Part model, mm, in its own coordinate system. Coordinates: 2 decimals unless noted, no trailing zeros. Loops run counter-clockwise (first coordinate to the right, second up) from the corner with the lowest first, then second, coordinate; pieces in that order, holes last. Notation, with made-up numbers: M -32,70 L 21,70 A30 cw 21,94 Z; hole C 9,36.5 d9. An arc over 180 degrees is marked long. Use a Markdown table: item, result. Add a question column.
1) Band-saw the part on C-C (x = -10.5). List the corners of the cut face in (y, z).
2) Band-saw the part on B-B (y = 0.5). List the corners of the cut face in (x, z), plus the area to 3 significant figures.
3) Pin check, flat tips, straight feed: pin 1 Ø1 at (y, z) = (0, 14.5) entering from +X; pin 2 Ø10 at (x, z) = (11, 5) entering from -Y; pin 3 Ø6 at (x, y) = (1, 8.5) entering from +Z. Stop position of each tip, or through.
4) Band-saw the part on A-A (z = 5). List the corners of the cut face in (x, y) (1 decimal).
5) Wall check: probe 1 along Y at (x, z) = (-1, 4); probe 2 along X at (y, z) = (-6, 3.5); probe 3 along Y at (x, z) = (-7.5, 13.25). Give the ranges that are in metal, low to high. Write a range as from..to.
6) Band-saw the part on D-D (z = 1.5). List the corners of the cut face in (x, y), plus the area to 3 significant figures.
Autodesk Fusion 360 part; units mm, degrees
sketch "草图1" plane through (0, 0, 0) normal (0, 1, 0) x (1, 0, 0)
  line L0 (0, -55) -> (0, 50) construction
  line L1 (-125, 0) -> (125, 0) construction
  line L2 (-31, 0) -> (20, 0)
  circle A0 centre (20, -1) radius 1
  arc A1 (-31.065, -5.889) -> (18.5199, -10.8983) centre (-3, 24) ccw
  line L3 (-31.6884, -4.6053) -> (-31.9962, -1.0872)
  line L4 (20.4052, -7.8422) -> (20.9962, -1.0872)
  line L5 (21, 0) -> (21, -0.6) construction
  line L6 (-32, 0) -> (-32, -0.7) construction
  line L7 (0, -17) -> (10, -17) construction
  arc A2 (-31, 0) -> (-31.9962, -1.0872) centre (-31, -1) ccw
  arc A3 (-31.6884, -4.6053) -> (-31.065, -5.889) centre (-29.696, -4.431) ccw
  arc A4 (-8, 0) -> (8, 0) centre (0, 0) ccw
  arc A5 (18.5199, -10.8983) -> (20.4052, -7.8422) centre (16.4204, -7.4936) ccw
  line L8 (0, -8) -> (0, 0)
  dimension "d1" = 16
  dimension "d2" = 2
  dimension "d3" = 2
  dimension "d4" = 5
  dimension "d5" = 5
  dimension "d6" = 8
  dimension "d7" = 4
  dimension "d8" = 21
  dimension "d9" = 53
  dimension "d10" = 41
  dimension "d11" = 17
  dimension "d12" = 24
  dimension "d13" = 24
extrude "拉伸1" add sketch "草图1" along normal mid plane 30
revolve "旋转1" cut sketch "草图1" angle 360 about axis through (0, 0, 55) along (0, 0, -1) contours L2 A4 L8 picked at (-0.3795, -5.3062)
sketch "草图2" plane through (0, 0, 0) normal (0, 0, 1) x (1, 0, 0)
  line L0 (-31, -15) -> (20, -15)
  line L1 (20, 15) -> (-31, 15)
  arc A0 (18.3234, 13.6051) -> (-20.6815, 12.7204) centre (1.1833, -91) ccw
  arc A1 (-20.6815, -12.7204) -> (18.3234, -13.6051) centre (1.1833, 91) ccw
  line L2 (20, 11.6314) -> (20, -11.6314)
  arc A2 (20, 11.6314) -> (18.3234, 13.6051) centre (18, 11.6314) ccw
  arc A3 (18.3234, -13.6051) -> (20, -11.6314) centre (18, -11.6314) ccw
  arc A4 (-20.6815, 12.7204) -> (-20.6815, -12.7204) centre (-18, 0) ccw
  line L3 (-31, 15) -> (-31, -15) construction
  line L4 (-40, 0) -> (31, 0) construction
  dimension "d17" = 2
  dimension "d18" = 2
  dimension "d19" = 13
  dimension "d20" = 106
  dimension "d21" = 106
extrude "拉伸2" cut sketch "草图2" along normal blind 35 keep common part
sketch "草图3" plane through (0, 0, 0) normal (1, 0, 0) x (0, 1, 0)
  line L0 (-15, 0) -> (15, 0)
  line L1 (15, 0) -> (13.8335, 13.3333)
  line L2 (-15, 0) -> (-13.8335, 13.3333)
  line L3 (0, 45) -> (0, -20) construction
  line L4 (-40, 0) -> (40, 0) construction
  arc A0 (12.4483, 15.0645) -> (-12.4483, 15.0645) centre (0, -24) ccw
  arc A1 (-12.4483, 15.0645) -> (-13.8335, 13.3333) centre (-11.8411, 13.159) ccw
  arc A2 (13.8335, 13.3333) -> (12.4483, 15.0645) centre (11.8411, 13.159) ccw
  line L5 (0, 17) -> (10, 17) construction
  dimension "d24" = 10
  dimension "d25" = 30
  dimension "d26" = 4
  dimension "d27" = 4
  dimension "d28" = 41
  dimension "d29" = 17
extrude "拉伸3" cut sketch "草图3" along normal mid plane 100 keep common part
Entries:
| question | item | result |
|---|---|---|
| 1 | outline | M -14.35,0 L 14.35,0 L 14.35,7.38 L 13.83,13.33 A2 ccw 12.45,15.06 A41 ccw 7.5,16.31 L -7.5,16.31 A41 ccw -12.45,15.06 A2 ccw -13.83,13.33 L -14.35,7.38 Z |
| 2 | outline | M -30.99,0 L -7.98,0 A7.98 cw 7.98,0 L 20,0 L 20,9.28 A4 ccw 18.52,10.9 A41 ccw -2.5,17 L -3.5,17 A41 ccw -30.99,5.96 Z |
| 2 | area | 618 mm2 |
| 3 | pin 1 | x = 12.39 |
| 3 | pin 2 | y = -14.84 |
| 3 | pin 3 | z = 16.63 |
| 4 | outline | M -20.7,-12.7 A106 ccw -8.4,-14.6 L 10.8,-14.6 A106 ccw 18.3,-13.6 A2 ccw 20,-11.6 L 20,11.6 A2 ccw 18.3,13.6 A106 ccw 10.8,14.6 L -8.4,14.6 A106 ccw -20.7,12.7 A13 ccw Z; hole C 0,0 d12.5 |
| 5 | probe 1 | -14.65..-6.86, 6.86..14.65 |
| 5 | probe 2 | -29.53..-3.97, 3.97..20 |
| 5 | probe 3 | -13.84..13.84 |
| 6 | outline | M -20.68,-12.72 A106 ccw -4.09,-14.87 L 6.46,-14.87 A106 ccw 18.32,-13.61 A2 ccw 20,-11.63 L 20,11.63 A2 ccw 18.32,13.61 A106 ccw 6.46,14.87 L -4.09,14.87 A106 ccw -20.68,12.72 A13 ccw Z; hole C 0,0 d15.72 |
| 6 | area | 1,170 mm2 |
